from build123d import *

# Parameters (mm, degrees)
SKETCH1_W                    = 48.1584
SKETCH1_H                    = 38.227
SKETCH1_R                    = 9.525
SKETCH1_R_2                  = 1.778
BASE_FLANGE1_DEPTH           = 1.016
EDGE_FLANGE1_STRIP_W         = 6.604
EDGE_FLANGE1_STRIP_H         = 1.016
EDGE_FLANGE1_STRIP_CUT_DEPTH = 48.1584
EDGE_FLANGE1_DEPTH           = 48.1584
EDGE_FLANGE1_START           = 1.016
EDGE_FLANGE1_PROFILE_W       = 48.1584
EDGE_FLANGE1_PROFILE_H       = 43.5102
EDGE_FLANGE1_PROFILE_R       = 4.73075
EDGE_FLANGE1_FLAT_DEPTH      = 1.016
CUT_EXTRUDE7_DEPTH           = 65.852611865
FILLET2_R                    = 7.62
FILLET3_R                    = 3.81


# Sheet-metal steps are written as plain solids
with BuildPart() as part:
    # Sketch1 → Base-Flange1 (new body)
    with BuildSketch(Plane(origin=(0, 0, 0), x_dir=(1, 0, 0), z_dir=(0, 1, 0))):
        Rectangle(SKETCH1_W, SKETCH1_H)
        with Locations(Location((0, 0, 0), (0, 0, 270))):
            Circle(SKETCH1_R, mode=Mode.SUBTRACT)
        with Locations(Location((13.470384182, -13.470384182, 0), (0, 0, 270))):
            Circle(SKETCH1_R_2, mode=Mode.SUBTRACT)
        with Locations(Location((13.470384182, 13.470384182, 0), (0, 0, 270))):
            Circle(SKETCH1_R_2, mode=Mode.SUBTRACT)
        with Locations(Location((-13.470384182, 13.470384182, 0), (0, 0, 90))):
            Circle(SKETCH1_R_2, mode=Mode.SUBTRACT)
        with Locations(Location((-13.470384182, -13.470384182, 0), (0, 0, 90))):
            Circle(SKETCH1_R_2, mode=Mode.SUBTRACT)
    extrude(amount=-BASE_FLANGE1_DEPTH)

    # Edge-Flange1 strip (across the edge) → Edge-Flange1 strip cut (cut)
    with BuildSketch(Plane(origin=(24.0792, 0, -19.1135), x_dir=(0, 0, 1), z_dir=(-1, 0, 0))):
        with Locations((-2.032, -0.508)):
            Rectangle(EDGE_FLANGE1_STRIP_W, EDGE_FLANGE1_STRIP_H)
    edge_flange1_strip_cut = extrude(amount=EDGE_FLANGE1_STRIP_CUT_DEPTH, mode=Mode.SUBTRACT)

    # Edge-Flange1 bend section (across the edge) → Edge-Flange1 (add)
    with BuildSketch(Plane(origin=(24.0792, 0, -19.1135), x_dir=(0, 0, 1), z_dir=(-1, 0, 0))):
        with BuildLine():
            Line((-1.016, 1.27), (0, 1.27))
            ThreePointArc((0, 1.27), (0.371974388, 0.371974388), (1.27, 0))
            Line((1.27, 0), (1.27, -1.016))
            ThreePointArc((1.27, -1.016), (-0.346446102, -0.346446102), (-1.016, 1.27))
        make_face()
    edge_flange1 = extrude(amount=EDGE_FLANGE1_DEPTH)

    # Edge-Flange1 profile (on flange) → Edge-Flange1 flat (add)
    with BuildSketch(Plane(origin=(0, 0, -19.1135), x_dir=(-1, 0, 0), z_dir=(0, 0, -1)).offset(EDGE_FLANGE1_START)):
        with Locations((0, 23.0251)):
            Rectangle(EDGE_FLANGE1_PROFILE_W, EDGE_FLANGE1_PROFILE_H)
        with Locations((-15.113, 35.814)):
            Circle(EDGE_FLANGE1_PROFILE_R, mode=Mode.SUBTRACT)
        with Locations((15.113, 35.814)):
            Circle(EDGE_FLANGE1_PROFILE_R, mode=Mode.SUBTRACT)
    edge_flange1_flat = extrude(amount=-EDGE_FLANGE1_FLAT_DEPTH)

    # Mirror1: Edge-Flange1 strip cut, Edge-Flange1, Edge-Flange1 flat across plane
    add(edge_flange1_strip_cut.mirror(Plane.XY), mode=Mode.SUBTRACT)
    add(edge_flange1.mirror(Plane.XY))
    add(edge_flange1_flat.mirror(Plane.XY))

    # Sketch11 → Cut-Extrude7 (cut, through all)
    with BuildSketch(Plane(origin=(0, 0, -20.1295), x_dir=(-1, 0, 0), z_dir=(0, 0, -1))):
        with BuildLine():
            Line((24.0792, 43.18), (24.0792, 44.7802))
            Line((24.0792, 44.7802), (-24.0792, 44.7802))
            Line((-24.0792, 44.7802), (-24.0792, 43.18))
            Line((-24.0792, 43.18), (-15.113, 43.18))
            ThreePointArc((-15.113, 43.18), (-9.90445145, 41.02254855), (-7.747, 35.814))
            Line((-7.747, 35.814), (7.747, 35.814))
            ThreePointArc((7.747, 35.814), (9.90445145, 41.02254855), (15.113, 43.18))
            Line((15.113, 43.18), (24.0792, 43.18))
        make_face()
    extrude(amount=-CUT_EXTRUDE7_DEPTH, mode=Mode.SUBTRACT)

    # Fillet2
    fillet2_edges = [part.edges().sort_by_distance(p)[0] for p in [
        (7.747, 35.814, -19.6215),
        (-7.747, 35.814, -19.6215),
        (7.747, 35.814, 19.6215),
        (-7.747, 35.814, 19.6215),
    ]]
    fillet(fillet2_edges, radius=FILLET2_R)

    # Fillet3
    fillet3_edges = [part.edges().sort_by_distance(p)[0] for p in [
        (-24.0792, 43.18, -19.6215),
        (24.0792, 43.18, -19.6215),
        (24.0792, 43.18, 19.6215),
        (-24.0792, 43.18, 19.6215),
    ]]
    fillet(fillet3_edges, radius=FILLET3_R)


solid = part.part
The listing builds one solid part. Answer for the finished solid, in the listing's coordinates (mm). A direction names the side the tool comes from. Give positions to 0.01 mm unless a question says otherwise; leave off trailing zeros. Write each loop counter-clockwise with the first axis right and the second up, starting at its lowest first coordinate (ties: lowest second). Pieces come first, ordered by that corner, then holes.
1) Section D-D (x = 7) is taken. Write down the section's boundary in (y, z).
2) A tool of negligible diameter and unlimited length cuts with its end or side. For faces 1 (the face through (0, 23, 19.114)), 2 (the face through (0.337, -0.364, -19.442)), 3 (the face through (6.03, 36.84, -19.61)), from which of +Z, -Z, +X, -X, +Y, -Y can it reach the whole face along a straight path? Write none if from no direction.
3) Section C-C (x = 0) is taken. Write down the section's boundary in (y, z) (1 decimal).
4) Section B-B (y = 21) is taken. Write down the section's boundary in (x, z), and give its area (3 significant figures).
5) Section A-A (z = 0) is taken. Write down the section's boundary in (x, y) (3 decimals).
6) Given P1, Ø4, axis at x = -13.47, z = -13.47, coming from the +Y side; P2, Ø4, axis at x = -13.47, z = 13.47, coming from the -Y side; P3, Ø1.1, axis at x = 0, z = -19.5, coming from the +Y side, each flat-ended and moving along its own axis, determine where each tip first touches the part or whether it passes through.
7) For a pull along X with two mould halves and no side action, classify faces 4 (the face through (-22.993, 42.034, 19.629)), 5 (the face through (-14.67, -0.5, -12.16)), 6 (the face through (24.079, -0.4, 0.1)) as pulls with the +X half, pulls with the -X half, needs draft (parallel to the pull), parting line crosses it, or undercut.
8) Find the intervals of material crossed by L1, parallel to Z at x = 12, y = 18; L2, parallel to Y at x = -10, z = 6.5; L3, parallel to X at y = -0.7, z = 0 (3 decimals), in increasing order.
Response:
1. outline: (-1.02, -17.84) arc R2.29 ccw to (1.27, -20.13) - (37.51, -20.13) - (37.51, -19.11) - (1.27, -19.11) arc R1.27 cw to (0, -17.84) - (0, -6.46) - (-1.02, -6.46) - close; (-1.02, 6.46) - (0, 6.46) - (0, 17.84) arc R1.27 cw to (1.27, 19.11) - (37.51, 19.11) - (37.51, 20.13) - (1.27, 20.13) arc R2.29 ccw to (-1.02, 17.84) - close
2. face 1: +X, -X, +Y
2. face 2: -Z, +X, -X, -Y
2. face 3: +Z, -Z, +Y
3. outline: (-1, -17.8) arc R2.3 ccw to (1.3, -20.1) - (35.8, -20.1) - (35.8, -19.1) - (1.3, -19.1) arc R1.3 cw to (0, -17.8) - (0, -9.5) - (-1, -9.5) - close; (-1, 9.5) - (0, 9.5) - (0, 17.8) arc R1.3 cw to (1.3, 19.1) - (35.8, 19.1) - (35.8, 20.1) - (1.3, 20.1) arc R2.3 ccw to (-1, 17.8) - close
4. outline: (-24.08, -20.13) - (24.08, -20.13) - (24.08, -19.11) - (-24.08, -19.11) - close; (-24.08, 19.11) - (24.08, 19.11) - (24.08, 20.13) - (-24.08, 20.13) - close
4. area: 97.9 mm2
5. outline: (-24.079, -1.016) - (-9.525, -1.016) - (-9.525, 0) - (-24.079, 0) - close; (9.525, -1.016) - (24.079, -1.016) - (24.079, 0) - (9.525, 0) - close
6. P1: stops at y = 0
6. P2: stops at y = -1.02
6. P3: stops at y = 35.81
7. face 4: pulls with the -X half
7. face 5: undercut
7. face 6: pulls with the +X half
8. L1: z = -20.13 to -19.11, 19.11 to 20.13
8. L2: y = -1.02 to 0
8. L3: x = -24.079 to -9.525, 9.525 to 24.079
